CAD build for the part. Positions are in the model's coordinates, mm. A direction names the side the tool comes from. Give positions to 0.01 mm unless a question says otherwise; leave off trailing zeros. Loops run counter-clockwise (first coordinate to the right, second up) from the corner with the lowest first, then second, coordinate; pieces in that order, holes last. Notation, with made-up numbers: (-9.5, -16) -> (7.5, -16) arc R18 ccw to (7.5, 13) -> close; hole circle Ø6 at (12.25, -18.5). An arc over 180 degrees is marked (long way). Use one line per item in the form item = value.
```python
from build123d import *

# Parameters (mm, degrees)
F0_R     = 15.875
F1_DEPTH = 1.778
F4_R     = 0.889
F5_DEPTH = 1.778
F7_DEPTH = 1.016


with BuildPart() as f1:
    # F0 (on Top) → F1 (new body)
    with BuildSketch(Plane.XY):
        Circle(F0_R)
    extrude(amount=-F1_DEPTH)

    # F4 (on face) → F5 (join)
    with BuildSketch(Plane.XY):
        with Locations((0, 10.658966)):
            Circle(F4_R)
        with Locations((-10.613078, 0)):
            Circle(F4_R)
        with Locations((0, -10.630104)):
            Circle(F4_R)
        with Locations((10.574064, 0)):
            Circle(F4_R)
    extrude(amount=F5_DEPTH)

    # F6 (on face) → F7 (join)
    with BuildSketch(Plane.XY):
        Polygon((-1.286464, 5.058349), (-1.454464, 5.058349), (-4.184472, 5.163349), (-4.205472, 3.231343), (-3.869471, 2.11834), (-3.848471, -0.212667), (-3.57547, -0.527667), (-3.55447, -1.51467), (-4.037472, -1.976672), (-3.827471, -2.543673), (-3.49147, -2.732674), (-3.61747, -6.407684), (4.509553, -6.533685), (4.446552, -5.630682), (3.69055, -5.06368), (3.41755, -4.517679), (2.262546, -3.929677), (2.283546, -3.026675), (2.409547, -2.438673), (2.136546, -2.039672), (2.367547, -1.55667), (2.766548, -1.43067), (2.871548, -1.157669), (2.955548, -0.065666), (4.341552, 1.173337), (4.950554, 1.92934), (6.714559, 2.769342), (6.567559, 3.063343), (4.929554, 3.210343), (4.635553, 3.525344), (3.816551, 3.168343), (2.976548, 3.756345), (2.619547, 3.672344), (1.737545, 4.281346), (1.170543, 4.323346), (0.687542, 4.176346), (-0.299461, 4.512347), (-0.677462, 5.68835), (-1.286464, 5.83535), align=None)
    extrude(amount=F7_DEPTH)


solid = f1.part
```
1. Cut at D-D, the plane x = -6. Write the cut outline in (y, z).
Result sheet:
outline = (-14.7, -1.78) -> (14.7, -1.78) -> (14.7, 0) -> (-14.7, 0) -> close
2. Mould opens along X. For faces 1 (the flat face through (2.913, -0.619, 0.501)), 2 (the cylindrical face through (-3.441, -15.497, -0.877)), 3 (the flat face through (0, 11, 1.778)), 4 (the flat face through (4.48, -6.09, 0.5)) say: pulls with the +X half, pulls with the -X half, needs draft (parallel to the pull), parting line crosses it, or undercut.
Result sheet:
face_1 = undercut
face_2 = parting line crosses it
face_3 = needs draft
face_4 = pulls with the +X half
3. Drill centre lines: line 1 (Z direction, x = 2.5, y = 2); line 2 (Z direction, x = -5, y = 13.5); line 3 (Y direction, x = -12.5, z = -1.1). Where is each one in solid material? Low to high.
Result sheet:
line_1 = -1.78 to 1.02
line_2 = -1.78 to 0
line_3 = -9.79 to 9.79
4. Cut at B-B, the plane z = -0.9. Write the cut outline in (x, y) (3 decimals).
Result sheet:
outline = circle Ø31.75 at (0, 0)
5. Tool access for faces 5 (the flat face through (3.4, 3.46, 0.5)), 6 (the cylindrical face through (-10.806, -0.868, 0.877)), 7 (the flat face through (-4.04, 2.68, 0.5)): list every direction of +Z, -Z, +X, -X, +Y, -Y with a clear straight run to the whole face (end or side of a thin tool).
Result sheet:
face_5 = +Z, +Y
face_6 = +Z
face_7 = +Z, -X
6. Drop flat-ended pins along their axis: P1, Ø5, axis at x = 7, y = 8.5, coming from the +Z side; P2, Ø9.5, axis at x = 7, y = -5, coming from the +Z side; P3, Ø1, axis at x = -6.5, z = 0, coming from the +Y side. Give the stop position or say it passes through.
Result sheet:
P1 = 0
P2 = 1.02
P3 = 14.7
7. Cut at A-A, the plane z = 1.4. Write the cut outline in (x, y), then the cut area to 3 significant figures.
Result sheet:
outline = circle Ø1.78 at (-10.61, 0); circle Ø1.78 at (0, -10.63); circle Ø1.78 at (0, 10.66); circle Ø1.78 at (10.57, 0)
area = 9.93 mm^2
8. Cut at C-C, the plane y = -3.5. Write the cut outline in (x, z), then the cut area to 3 significant figures.
Result sheet:
outline = (-15.48, -1.78) -> (15.48, -1.78) -> (15.48, 0) -> (2.27, 0) -> (2.27, 1.02) -> (-3.52, 1.02) -> (-3.52, 0) -> (-15.48, 0) -> close
area = 60.9 mm^2
